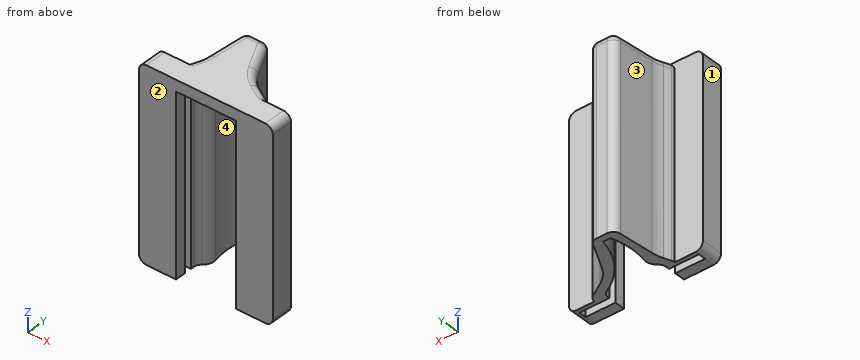
```python
from build123d import *

# Parameters (mm, degrees)
EXTRUSION1_DEPTH = 24
EXTRUSION2_START = 1.5
EXTRUSION2_DEPTH = 1.5
CONG_1_R         = 1


with BuildPart() as part:
    # Esquisse1 → Extrusion1 (new body)
    with BuildSketch(Plane.XY):
        with BuildLine():
            Line((-5.185390739, 1.525025478), (-5.185390739, 1.576014862))
            ThreePointArc((-5.185390739, 1.576014862), (-5.167721774, 1.763166505), (-5.115339265, 1.943704595))
            Line((-5.115339265, 1.943704595), (-4.776128633, 2.801624733))
            ThreePointArc((-4.776128633, 2.801624733), (-4.554638642, 3.512645897), (-4.441213812, 4.248678315))
            Line((-4.441213812, 4.248678315), (-4.072373491, 8.946086961))
            ThreePointArc((-4.072373491, 8.946086961), (-3.754309066, 9.602069144), (-3.075442001, 9.867807945))
            Line((-3.075442001, 9.867807945), (-1.611111903, 9.867807945))
            ThreePointArc((-1.611111903, 9.867807945), (-1.089661402, 9.721089477), (-0.721223737, 9.323986693))
            Line((-0.721223737, 9.323986693), (1.201547539, 5.573151281))
            ThreePointArc((1.201547539, 5.573151281), (2.003498303, 4.434130377), (3.08856632, 3.560562379))
            Line((3.08856632, 3.560562379), (5.060428728, 2.383722007))
            ThreePointArc((5.060428728, 2.383722007), (5.417566192, 2.018743813), (5.547944317, 1.525025478))
            Line((5.547944317, 1.525025478), (7.966203889, 1.525025478))
            Line((7.966203889, 1.525025478), (8.966203889, 1.525025478))
            Line((8.966203889, 1.525025478), (8.966203889, -1.412448643))
            Line((8.966203889, -1.412448643), (7.966203889, -1.412448643))
            Line((7.966203889, -1.412448643), (4, -1.412448643))
            Line((4, -1.412448643), (4, 0))
            Line((4, 0), (8, 0))
            Line((8, 0), (8, 1))
            Line((8, 1), (4, 1))
            Line((4, 1), (4, 1.202041029))
            ThreePointArc((4, 1.202041029), (3.852802865, 1.724273997), (3.454545455, 2.092764572))
            ThreePointArc((3.454545455, 2.092764572), (0.040046913, 4.946972092), (-1.797958971, 9))
            Line((-1.797958971, 9), (-2.797958971, 9))
            ThreePointArc((-2.797958971, 9), (-3.257790087, 6.426670848), (-3.034989317, 3.822092686))
            ThreePointArc((-3.034989317, 3.822092686), (-3.093760184, 2.977994654), (-3.6, 2.3))
            ThreePointArc((-3.6, 2.3), (-3.894427191, 1.947213595), (-4, 1.5))
            Line((-4, 1.5), (-4, 1))
            Line((-4, 1), (-8, 1))
            Line((-8, 1), (-8, 0))
            Line((-8, 0), (-4, 0))
            Line((-4, 0), (-4, -1.412448643))
            Line((-4, -1.412448643), (-7.966203889, -1.412448643))
            Line((-7.966203889, -1.412448643), (-8.966203889, -1.412448643))
            Line((-8.966203889, -1.412448643), (-8.966203889, 1.525025478))
            Line((-8.966203889, 1.525025478), (-7.966203889, 1.525025478))
            Line((-7.966203889, 1.525025478), (-5.185390739, 1.525025478))
        make_face()
    extrude(amount=-EXTRUSION1_DEPTH)

    # Esquisse2 → Extrusion2 (add)
    with BuildSketch(Plane.XY.offset(EXTRUSION2_START)):
        with BuildLine():
            Line((-4, -1.412448643), (4, -1.412448643))
            Line((4, -1.412448643), (8.966203889, -1.412448643))
            Line((8.966203889, -1.412448643), (8.966203889, 1.525025478))
            Line((8.966203889, 1.525025478), (5.547944317, 1.525025478))
            ThreePointArc((5.547944317, 1.525025478), (5.417566192, 2.018743813), (5.060428728, 2.383722007))
            Line((5.060428728, 2.383722007), (3.08856632, 3.560562379))
            ThreePointArc((3.08856632, 3.560562379), (2.003498303, 4.434130377), (1.201547539, 5.573151281))
            Line((1.201547539, 5.573151281), (-0.721223737, 9.323986693))
            ThreePointArc((-0.721223737, 9.323986693), (-1.089661402, 9.721089477), (-1.611111903, 9.867807945))
            Line((-1.611111903, 9.867807945), (-3.075442001, 9.867807945))
            ThreePointArc((-3.075442001, 9.867807945), (-3.754309066, 9.602069144), (-4.072373491, 8.946086961))
            Line((-4.072373491, 8.946086961), (-4.441213812, 4.248678315))
            ThreePointArc((-4.441213812, 4.248678315), (-4.554638642, 3.512645897), (-4.776128633, 2.801624733))
            Line((-4.776128633, 2.801624733), (-5.115339265, 1.943704595))
            ThreePointArc((-5.115339265, 1.943704595), (-5.167721774, 1.763166505), (-5.185390739, 1.576014862))
            Line((-5.185390739, 1.576014862), (-5.185390739, 1.525025478))
            Line((-5.185390739, 1.525025478), (-8.966203889, 1.525025478))
            Line((-8.966203889, 1.525025478), (-8.966203889, -1.412448643))
            Line((-8.966203889, -1.412448643), (-4, -1.412448643))
        make_face()
    extrude(amount=-EXTRUSION2_DEPTH)

    # Congé1
    # the kernel refuses this fillet: 1 mm, written as the material it takes off along each edge
    with BuildSketch(Plane(origin=(4.547944317, 1.525025478, 1.5), x_dir=(1, 0, 0), z_dir=(0, -1, 0))) as cong_1_piece_1:
        with BuildLine():
            CenterArc((1 - CONG_1_R, -CONG_1_R), CONG_1_R, 0, 90)
            Line((1, -CONG_1_R), (1, 0))
            Line((1, 0), (1 - CONG_1_R, 0))
        make_face()
    revolve(axis=Axis((4.547944317, 1.525025478, 1.5), (0, 0, 1)), revolution_arc=59.170542775, mode=Mode.SUBTRACT)
    with BuildSketch(Plane(origin=(5.060428728, 2.383722007, 1.5), x_dir=(-0.5124844104197742, -0.8586965290931928, 0), z_dir=(-0.8586965290931928, 0.5124844104197742, 0))) as cong_1_piece_2:
        with BuildLine():
            CenterArc((CONG_1_R, -CONG_1_R), CONG_1_R, 90, 90)
            Line((0, -CONG_1_R), (0, 0))
            Line((0, 0), (CONG_1_R, 0))
        make_face()
    extrude(amount=2.29634375, mode=Mode.SUBTRACT)
    with BuildSketch(Plane(origin=(5.650988372, 7.854045025, 1.5), x_dir=(-0.512484410419771, -0.8586965290931947, 0), z_dir=(0.8586965290931947, -0.512484410419771, 0))) as cong_1_piece_3:
        with BuildLine():
            CenterArc((5 + CONG_1_R, CONG_1_R), CONG_1_R, 180, 90)
            Line((5, CONG_1_R), (5, 0))
            Line((5, 0), (5 + CONG_1_R, 0))
        make_face()
    revolve(axis=Axis((5.650988372, 7.854045025, 1.5), (0, 0, -1)), revolution_arc=32.029740096, mode=Mode.SUBTRACT)
    with BuildSketch(Plane(origin=(1.201547539, 5.573151281, 1.5), x_dir=(-0.8898881666598102, -0.45617874878038983, 0), z_dir=(-0.45617874878038983, 0.8898881666598102, 0))) as cong_1_piece_4:
        with BuildLine():
            CenterArc((CONG_1_R, -CONG_1_R), CONG_1_R, 90, 90)
            Line((0, -CONG_1_R), (0, 0))
            Line((0, 0), (CONG_1_R, 0))
        make_face()
    extrude(amount=4.214951443, mode=Mode.SUBTRACT)
    with BuildSketch(Plane(origin=(-1.611111903, 8.867807945, 1.5), x_dir=(0.8898881666598123, 0.4561787487803857, 0), z_dir=(0.4561787487803857, -0.8898881666598123, 0))) as cong_1_piece_5:
        with BuildLine():
            CenterArc((1 - CONG_1_R, -CONG_1_R), CONG_1_R, 0, 90)
            Line((1, -CONG_1_R), (1, 0))
            Line((1, 0), (1 - CONG_1_R, 0))
        make_face()
    revolve(axis=Axis((-1.611111903, 8.867807945, 1.5), (0, 0, 1)), revolution_arc=62.859197321, mode=Mode.SUBTRACT)
    with BuildSketch(Plane(origin=(-5.185390739, 1.576014862, 1.5), x_dir=(1, 0, 0), z_dir=(0, -1, 0))) as cong_1_piece_6:
        with BuildLine():
            CenterArc((CONG_1_R, -CONG_1_R), CONG_1_R, 90, 90)
            Line((0, -CONG_1_R), (0, 0))
            Line((0, 0), (CONG_1_R, 0))
        make_face()
    extrude(amount=0.050989385, mode=Mode.SUBTRACT)
    with BuildSketch(Plane(origin=(-4.185390739, 1.576014862, 1.5), x_dir=(-0.9299485255595245, 0.3676897330762265, 0), z_dir=(0.3676897330762265, 0.9299485255595245, 0))) as cong_1_piece_7:
        with BuildLine():
            CenterArc((1 - CONG_1_R, -CONG_1_R), CONG_1_R, 0, 90)
            Line((1, -CONG_1_R), (1, 0))
            Line((1, 0), (1 - CONG_1_R, 0))
        make_face()
    revolve(axis=Axis((-4.185390739, 1.576014862, 1.5), (0, 0, 1)), revolution_arc=21.573207514, mode=Mode.SUBTRACT)
    with BuildSketch(Plane(origin=(-4.776128633, 2.801624733, 1.5), x_dir=(0.9299485255595272, -0.3676897330762192, 0), z_dir=(-0.3676897330762192, -0.9299485255595272, 0))) as cong_1_piece_8:
        with BuildLine():
            CenterArc((CONG_1_R, -CONG_1_R), CONG_1_R, 90, 90)
            Line((0, -CONG_1_R), (0, 0))
            Line((0, 0), (CONG_1_R, 0))
        make_face()
    extrude(amount=0.922545834, mode=Mode.SUBTRACT)
    with BuildSketch(Plane(origin=(-9.425871261, 4.640073399, 1.5), x_dir=(0.9969314898888016, -0.07827901678032455, 0), z_dir=(0.07827901678032455, 0.9969314898888016, 0))) as cong_1_piece_9:
        with BuildLine():
            CenterArc((5 + CONG_1_R, CONG_1_R), CONG_1_R, 180, 90)
            Line((5, CONG_1_R), (5, 0))
            Line((5, 0), (5 + CONG_1_R, 0))
        make_face()
    revolve(axis=Axis((-9.425871261, 4.640073399, 1.5), (0, 0, -1)), revolution_arc=17.083557109, mode=Mode.SUBTRACT)
    with BuildSketch(Plane(origin=(-4.072373491, 8.946086961, 1.5), x_dir=(0.9969314898888012, -0.07827901678032895, 0), z_dir=(-0.07827901678032895, -0.9969314898888012, 0))) as cong_1_piece_10:
        with BuildLine():
            CenterArc((CONG_1_R, -CONG_1_R), CONG_1_R, 90, 90)
            Line((0, -CONG_1_R), (0, 0))
            Line((0, 0), (CONG_1_R, 0))
        make_face()
    extrude(amount=4.711867058, mode=Mode.SUBTRACT)
    with BuildSketch(Plane(origin=(-3.075442001, 8.867807945, 1.5), x_dir=(0, 1, 0), z_dir=(1, 0, 0))) as cong_1_piece_11:
        with BuildLine():
            CenterArc((1 - CONG_1_R, -CONG_1_R), CONG_1_R, 0, 90)
            Line((1, -CONG_1_R), (1, 0))
            Line((1, 0), (1 - CONG_1_R, 0))
        make_face()
    revolve(axis=Axis((-3.075442001, 8.867807945, 1.5), (0, 0, 1)), revolution_arc=85.510349595, mode=Mode.SUBTRACT)
    with BuildSketch(Plane(origin=(-8.966203889, -3.912448643, -24), x_dir=(1, 0, 0), z_dir=(0, 1, 0)), Plane(origin=(8.966203889, 4.025025478, -24), x_dir=(-1, 0, 0), z_dir=(0, -1, 0)), Plane(origin=(-8.966203889, 4.025025478, 1.5), x_dir=(1, 0, 0), z_dir=(0, -1, 0))) as cong_1_piece_12:
        with BuildLine():
            CenterArc((CONG_1_R, -CONG_1_R), CONG_1_R, 90, 90)
            Line((0, -CONG_1_R), (0, 0))
            Line((0, 0), (CONG_1_R, 0))
        make_face()
    extrude(amount=7.937474121, mode=Mode.SUBTRACT)
    with BuildSketch(Plane(origin=(8.966203889, -3.912448643, 1.5), x_dir=(0, 0, -1), z_dir=(0, 1, 0))) as cong_1_piece_13:
        with BuildLine():
            CenterArc((CONG_1_R, CONG_1_R), CONG_1_R, 180, 90)
            Line((0, CONG_1_R), (0, 0))
            Line((0, 0), (CONG_1_R, 0))
        make_face()
    extrude(amount=7.937474121, mode=Mode.SUBTRACT)
    with BuildSketch(Plane(origin=(-1.611111903, 9.867807945, 1.5), x_dir=(0, -1, 0), z_dir=(-1, 0, 0))) as cong_1_piece_14:
        with BuildLine():
            CenterArc((CONG_1_R, -CONG_1_R), CONG_1_R, 90, 90)
            Line((0, -CONG_1_R), (0, 0))
            Line((0, 0), (CONG_1_R, 0))
        make_face()
    extrude(amount=1.464330098, mode=Mode.SUBTRACT)


solid = part.part
```
Could you check a few things on this model? Use its own coordinates, in mm. Face numbers are marked on the shaded views. Round coordinates to 2 decimals unless told otherwise and drop trailing zeros. Write each loop counter-clockwise with the first axis right and the second up, starting at its lowest first coordinate (ties: lowest second). Pieces come first, ordered by that corner, then holes. Notation, with made-up numbers: M 84,-3 L 90,-3 A18 cw 90,4 Z; hole C -35,66 d5. An arc over 180 degrees is marked long. Write each question's results on one line, items separated by ' | '. Start each with the question number.
1. I need wall thicknesses on L1, parallel to Y at x = -7, z = -8.25; L2, parallel to X at y = 6.5, z = -5.25; L3, parallel to X at y = 3.5, z = -9.5. Which ranges of each line are inside material? Lowest first, please. Write a range as from..to.
2. Thinking about a two-plate mould opening in Y: for the marked faces 1, 2, 3 and 4, which applies, +Y half, -Y half, draft (parallel to the pull), parting line (faces both ways), or undercut?
3. Imagine slicing it at A-A on x = -7.5. List the corners of the cut face in (y, z) for me.
4. I'm going to push flat-ended pins straight in: pin 1 Ø3.5 at (x, z) = (6, -17) entering from +Y; pin 2 Ø4 at (x, z) = (-5.5, -11.5) entering from +Y; pin 3 Ø10 at (x, z) = (7, -8) entering from +Y. Where does each tip first touch, or does it pass through?
Result sheet:
1) L1: y = -1.41..0, 1..1.53 | L2: x = -4.26..-3.25, -0.93..0.73 | L3: x = -4.56..-3, 1.39..3.19
2) face 1: draft | face 2: -Y half | face 3: +Y half | face 4: undercut
3) outline: M -1.41,-24 L 0,-24 L 0,0 L 1,0 L 1,-24 L 1.53,-24 L 1.53,1.5 L -1.41,1.5 Z
4) pin 1: stops at y = 2.87 | pin 2: stops at y = 9.77 | pin 3: stops at y = 4.44
